Read the model definition and answer for the solid it produces. Units are mm, in the model's axes. A direction names the side the tool comes from. Give positions to 0.01 mm unless a question says otherwise; leave off trailing zeros. Write each loop counter-clockwise with the first axis right and the second up, starting at its lowest first coordinate (ties: lowest second). Pieces come first, ordered by that corner, then holes.
```python
from build123d import *

# Parameters (mm, degrees)
SKETCH1_R                   = 18.288
BOSS_EXTRUDE1_DEPTH         = 19.05
SKETCH3_R                   = 13.208
CUT_EXTRUDE1_DEPTH          = 16.51
CUT_EXTRUDE2_REACH          = 32.684
SKETCH6_R                   = 10.668
SKETCH10_W                  = 6.858
SKETCH10_H                  = 2.794
CUT_EXTRUDE3_DEPTH          = 11.63828
CIRPATTERN1_COUNT           = 3
CIRPATTERN2_COUNT           = 3
SKETCH15_W                  = 19.05
SKETCH15_H                  = 17.526
BOSS_EXTRUDE3_DEPTH         = 15.24
SKETCH16_W                  = 11.43
SKETCH16_H                  = 5.842
CUT_EXTRUDE4_DEPTH          = 39.824629185
CHAMFER1_SIZE               = 8.129699408
CHAMFER1_SIZE_2             = 5.08
F_1_4_CLEARANCE_HOLE1_D     = 6.7564
F_1_4_CLEARANCE_HOLE1_DEPTH = 3.448428068


with BuildPart() as part:
    # Sketch1 → Boss-Extrude1 (new body)
    with BuildSketch(Plane.XY):
        with Locations(Location((0, 0, 0), (0, 0, 180))):
            Circle(SKETCH1_R)
    extrude(amount=BOSS_EXTRUDE1_DEPTH)

    # Sketch3 → Cut-Extrude1 (cut)
    with BuildSketch(Plane.XY.offset(19.05)):
        Circle(SKETCH3_R)
    extrude(amount=-CUT_EXTRUDE1_DEPTH, mode=Mode.SUBTRACT)

    # Sketch6 → Cut-Extrude2 (cut, up to next)
    with BuildSketch(Plane.XY.offset(2.54), mode=Mode.PRIVATE) as cut_extrude2_sk1:
        Circle(SKETCH6_R)
    cut_extrude2_tool1 = extrude(cut_extrude2_sk1.sketch, amount=-CUT_EXTRUDE2_REACH, mode=Mode.PRIVATE) & part.part
    add(cut_extrude2_tool1.solids().sort_by_distance((0, 0, 2.54))[0], mode=Mode.SUBTRACT)

    # Sketch10 → Cut-Extrude3 (cut)
    with BuildSketch(Plane.XY.offset(19.05)):
        with Locations((0, 15.526400014)):
            Rectangle(SKETCH10_W, SKETCH10_H)
    cut_extrude3 = extrude(amount=-CUT_EXTRUDE3_DEPTH, mode=Mode.SUBTRACT)

    # CirPattern1: Cut-Extrude3 ×3 about axis
    cirpattern1_axis = Axis((0, 0, 0), (0, 0, 1))
    for i in range(1, CIRPATTERN1_COUNT):
        add(cut_extrude3.rotate(cirpattern1_axis, i * 360 / CIRPATTERN1_COUNT), mode=Mode.SUBTRACT)

    # Sketch13 → #4 Clearance Hole1 (revolve, cut)
    with BuildSketch(Plane(origin=(0, 10.16, 11.039220548), x_dir=(0, 0, -1), z_dir=(1, 0, 0))):
        Polygon((0, 0), (0, 13.680574487), (1.63195, 12.7), (1.63195, 0), align=None)
    f_4_clearance_hole1 = revolve(axis=Axis((0, 3.81, 11.039220548), (0, 1, 0)), mode=Mode.SUBTRACT)

    # CirPattern2: #4 Clearance Hole1 ×3 about axis
    cirpattern2_axis = Axis((0, 0, 19.05), (0, 0, -1))
    for i in range(1, CIRPATTERN2_COUNT):
        add(f_4_clearance_hole1.rotate(cirpattern2_axis, i * 360 / CIRPATTERN2_COUNT), mode=Mode.SUBTRACT)

    # Sketch15 → Boss-Extrude3 (add)
    with BuildSketch(Plane(origin=(0, -13.716, 0), x_dir=(1, 0, 0), z_dir=(0, 1, 0))):
        with Locations((0, -9.525)):
            Rectangle(SKETCH15_W, SKETCH15_H)
    extrude(amount=-BOSS_EXTRUDE3_DEPTH)

    # Sketch16 → Cut-Extrude4 (cut, through all)
    with BuildSketch(Plane.XY.offset(18.288)):
        with Locations((0, -22.586571932)):
            Rectangle(SKETCH16_W, SKETCH16_H)
    extrude(amount=-CUT_EXTRUDE4_DEPTH, mode=Mode.SUBTRACT)

    # Chamfer1
    # the kernel refuses this chamfer: 8.129699408, 5.08 mm, written as the material it takes off along each edge
    with BuildSketch(Plane(origin=(-30.543101737, -28.956, 0.762), x_dir=(0, 0.9997899140358644, -0.020497019104217945), z_dir=(1, 0, 0))) as chamfer1_piece_1:
        Polygon((CHAMFER1_SIZE * 0.999789913978, CHAMFER1_SIZE * 0.020497019103), (-CHAMFER1_SIZE_2 * 0.0204970191042, CHAMFER1_SIZE_2 * 0.999789914036), (0, 0), align=None)
    extrude(amount=61.086203475, mode=Mode.SUBTRACT)

    # 1/4 Clearance Hole1
    with Locations(Plane(origin=(0, -28.956, 0), x_dir=(-1, 0, 0), z_dir=(0, -1, 0))):
        with Locations((0, -12.021417661)):
            Hole(F_1_4_CLEARANCE_HOLE1_D / 2, depth=F_1_4_CLEARANCE_HOLE1_DEPTH)


solid = part.part
```
Item 1: Section D-D (x = 0) is taken. Give the number of separate pieces and of enclosed holes in the cut face, and give its area (3 significant figures).
Result set:
separate pieces: 6
enclosed holes: 0
area: 214 mm2
Item 2: Each of these flat-tipped pins is pushed along its axis until it touches: pin 1 Ø6 at (y, z) = (-19, 4.5) entering from +X (3 decimals); pin 2 Ø4.5 at (y, z) = (-23, 13) entering from -X (3 decimals); pin 3 Ø2 at (x, z) = (9.5, 10) entering from +Y. Where does it stop, or does it pass through?
Result set:
pin 1: stops at x = 9.525
pin 2: stops at x = -9.525
pin 3: stops at y = 16.19
Item 3: Determine the mould class of faces 4 (the flat face through (9.525, -22, 10)), 5 (the flat face through (-3.429, 16, 13)), 6 (the cylindrical face through (0.625, 13.611, 9.532)), 7 (the flat face through (6, 12, 19.05)) for opening direction X: pulls with the +X half, pulls with the -X half, needs draft (parallel to the pull), parting line crosses it, or undercut.
Result set:
face 4: pulls with the +X half
face 5: undercut
face 6: undercut
face 7: needs draft
Item 4: Which of the six approach directions +Z, -Z, +X, -X, +Y, -Y give full straight-line access (tool end or side, diameter ignored) to faces 1 (the flat face through (-5.715, -23, 10)), 2 (the cylindrical face through (12.598, 3.967, 10.911)), 3 (the flat face through (-8, 8, 0))?
Result set:
face 1: +Z, -Z
face 2: +Z
face 3: -Z, +X, -X, +Y, -Y
Item 5: Section C-C (x = 9) is taken. Write down the section's boundary in (y, z), and give its area (3 significant figures).
Result set:
outline: (-28.96, 5.84) - (-20.83, 0.76) - (-15.92, 0.76) - (-15.92, 0) - (-5.73, 0) - (-5.73, 2.54) - (-9.67, 2.54) - (-9.67, 19.05) - (-15.92, 19.05) - (-15.92, 18.29) - (-28.96, 18.29) - close; (5.73, 0) - (15.92, 0) - (15.92, 19.05) - (9.67, 19.05) - (9.67, 2.54) - (5.73, 2.54) - close
area: 466 mm2
Item 6: Section B-B (z = 17.25) is taken. Write down the section's boundary in (x, y) (3 decimals).
Result set:
outline: (-9.525, -28.956) - (9.525, -28.956) - (9.525, -15.612) arc R18.288 ccw (long way) to (-9.525, -15.612) - close; hole (-16.371, -5.492) - (-12.942, -11.431) - (-10.522, -10.034) - (-13.951, -4.095) - close; hole circle Ø26.416 at (0, 0); hole (-5.715, -25.508) - (5.715, -25.508) - (5.715, -19.666) - (-5.715, -19.666) - close; hole (-3.429, 14.129) - (3.429, 14.129) - (3.429, 16.923) - (-3.429, 16.923) - close; hole (10.522, -10.034) - (12.942, -11.431) - (16.371, -5.492) - (13.951, -4.095) - close
Item 7: Section A-A (y = 0) is taken. Write down the section's boundary in (x, z), and give its area (3 significant figures).
Result set:
outline: (-18.29, 0) - (-10.67, 0) - (-10.67, 2.54) - (-13.21, 2.54) - (-13.21, 19.05) - (-18.29, 19.05) - close; (10.67, 0) - (18.29, 0) - (18.29, 19.05) - (13.21, 19.05) - (13.21, 2.54) - (10.67, 2.54) - close
area: 206 mm2
Item 8: Find the intervals of material crossed by line 1 along Y through (x, z) = (0, 14.25); line 2 along Y through (x, z) = (0, 1.9); line 3 along Y through (x, z) = (-5.5, 17), in increasing order.
Result set:
line 1: y = -19.67 to -13.21, 13.21 to 14.13, 16.92 to 18.29
line 2: y = -19.67 to -10.67, 10.67 to 18.29
line 3: y = -28.96 to -25.51, -19.67 to -12.01, 12.01 to 17.44
